```python
from build123d import *

# Parameters (mm, degrees)
SKETCH1_W           = 90
SKETCH1_H           = 50
BOSS_EXTRUDE1_DEPTH = 40
SKETCH21_R          = 5
CUT_EXTRUDE10_DEPTH = 40
SKETCH22_W          = 40
SKETCH22_H          = 13.4
CUT_EXTRUDE11_DEPTH = 9
SKETCH24_W          = 24
SKETCH24_H          = 13.4
CUT_EXTRUDE12_DEPTH = 31
SKETCH25_R          = 1.1
CUT_EXTRUDE13_DEPTH = 31
SKETCH31_W          = 25
SKETCH31_H          = 40
BOSS_EXTRUDE2_DEPTH = 50
SKETCH32_R          = 10
CUT_EXTRUDE15_DEPTH = 25
CHAMFER1_SIZE       = 10
CUT_EXTRUDE16_REACH = 142.357
SKETCH35_W          = 15
SKETCH35_H          = 20
SKETCH36_W          = 12
SKETCH36_H          = 12
SKETCH36_R          = 3.5
BOSS_EXTRUDE3_DEPTH = 10


with BuildPart() as part:
    # Sketch1 → Boss-Extrude1 (new body)
    with BuildSketch(Plane.XY):
        with Locations((-45, 25)):
            Rectangle(SKETCH1_W, SKETCH1_H)
    extrude(amount=BOSS_EXTRUDE1_DEPTH)

    # Sketch21 → Cut-Extrude10 (cut)
    with BuildSketch(Plane.XY.offset(40)):
        with Locations((-25, 25)):
            Circle(SKETCH21_R)
        with BuildLine():
            Line((-25, 30), (-30, 30))
            Line((-30, 30), (-30, 25))
            ThreePointArc((-30, 25), (-28.535533906, 28.535533906), (-25, 30))
        make_face()
        with BuildLine():
            ThreePointArc((-25, 20), (-28.535533906, 21.464466094), (-30, 25))
            Line((-30, 25), (-30, 20))
            Line((-30, 20), (-25, 20))
        make_face()
        with BuildLine():
            Line((-20, 20), (-20, 25))
            ThreePointArc((-20, 25), (-21.464466094, 21.464466094), (-25, 20))
            Line((-25, 20), (-20, 20))
        make_face()
        with BuildLine():
            Line((-20, 30), (-25, 30))
            ThreePointArc((-25, 30), (-21.464466094, 28.535533906), (-20, 25))
            Line((-20, 25), (-20, 30))
        make_face()
    extrude(amount=-CUT_EXTRUDE10_DEPTH, mode=Mode.SUBTRACT)

    # Sketch22 → Cut-Extrude11 (cut)
    with BuildSketch(Plane.XY.offset(40)):
        with Locations((-59.75, 25)):
            Rectangle(SKETCH22_W, SKETCH22_H)
    extrude(amount=-CUT_EXTRUDE11_DEPTH, mode=Mode.SUBTRACT)

    # Sketch24 → Cut-Extrude12 (cut)
    with BuildSketch(Plane.XY.offset(31)):
        with Locations((-59.75, 25)):
            Rectangle(SKETCH24_W, SKETCH24_H)
    extrude(amount=-CUT_EXTRUDE12_DEPTH, mode=Mode.SUBTRACT)

    # Sketch25 → Cut-Extrude13 (cut)
    with BuildSketch(Plane.XY.offset(31)):
        with Locations((-73.25, 25)):
            Circle(SKETCH25_R)
        with Locations((-46.25, 25)):
            Circle(SKETCH25_R)
    extrude(amount=-CUT_EXTRUDE13_DEPTH, mode=Mode.SUBTRACT)

    # Sketch31 → Boss-Extrude2 (add)
    with BuildSketch(Plane(origin=(0, 50, 0), x_dir=(1, 0, 0), z_dir=(0, 1, 0))):
        with Locations((-77.5, -20)):
            Rectangle(SKETCH31_W, SKETCH31_H)
    extrude(amount=BOSS_EXTRUDE2_DEPTH)

    # Sketch32 → Cut-Extrude15 (cut)
    with BuildSketch(Plane(origin=(-65, 0, 0), x_dir=(0, 0, -1), z_dir=(1, 0, 0))):
        with BuildLine():
            ThreePointArc((-40, 80), (-34.142135624, 94.142135624), (-20, 100))
            Line((-20, 100), (-40, 100))
            Line((-40, 100), (-40, 80))
        make_face()
        with BuildLine():
            ThreePointArc((-20, 100), (-5.857864376, 94.142135624), (0, 80))
            Line((0, 80), (0, 100))
            Line((0, 100), (-20, 100))
        make_face()
        with Locations((-20, 80)):
            Circle(SKETCH32_R)
    extrude(amount=-CUT_EXTRUDE15_DEPTH, mode=Mode.SUBTRACT)

    # Chamfer1
    chamfer1_edges = [part.edges().sort_by_distance(p)[0] for p in [
        (-65, 50, 20),
        (0, 50, 20),
        (0, 0, 20),
        (-90, 0, 20),
    ]]
    chamfer(chamfer1_edges, length=CHAMFER1_SIZE)

    # Cut-Extrude16: up to this face of the body (flat: up to its plane)
    cut_extrude16_end = Plane(part.part.faces().sort_by_distance((-47.75, 25, 15.5))[0])
    # Sketch35 → Cut-Extrude16 (cut, up to the picked face)
    with BuildSketch(Plane.ZY.offset(90), mode=Mode.PRIVATE) as cut_extrude16_sk1:
        with Locations((14.686432503, 25)):
            Rectangle(SKETCH35_W, SKETCH35_H)
    cut_extrude16_tool1 = split(extrude(cut_extrude16_sk1.sketch, amount=-CUT_EXTRUDE16_REACH, mode=Mode.PRIVATE), bisect_by=cut_extrude16_end, keep=Keep.BOTH, mode=Mode.PRIVATE)
    add(cut_extrude16_tool1.solids().sort_by(Axis((-90, 25, 14.686433), (1, 0, 0)))[0], mode=Mode.SUBTRACT)

    # Sketch36 → Boss-Extrude3 (add)
    # profile 1 of 2: a face of its own
    with BuildSketch(Plane.XY.offset(40)):
        with Locations((-65, -6)):
            Rectangle(SKETCH36_W, SKETCH36_H)
        with Locations((-65, -6)):
            Circle(SKETCH36_R, mode=Mode.SUBTRACT)
    # profile 2 of 2: a face of its own
    with BuildSketch(Plane.XY.offset(40)):
        with Locations((-25, -6)):
            Rectangle(SKETCH36_W, SKETCH36_H)
        with Locations((-25, -6)):
            Circle(SKETCH36_R, mode=Mode.SUBTRACT)
    extrude(amount=-BOSS_EXTRUDE3_DEPTH)


solid = part.part
```
Work out the finished part from the listing and answer in its coordinate system (mm). A direction names the side the tool comes from. Coordinates: 2 decimals unless noted, no trailing zeros. Write each loop counter-clockwise with the first axis right and the second up, starting at its lowest first coordinate (ties: lowest second). Pieces come first, ordered by that corner, then holes.
Q1. Determine the mould class of faces 1 (the face through (-47.75, 25, 16)), 2 (the face through (-85, 5, 20)), 3 (the face through (-25, -12, 35)) for opening direction X: released by +X, released by -X, zero draft, split by the parting line, or undercut.
Q2. Find the intervals of material crossed by line 1 (Y direction, x = -72, z = 20); line 2 (Y direction, x = -22, z = 14); line 3 (Y direction, x = -54.5, z = 23), in increasing order.
Q3. Each of these flat-tipped pins is pushed along its axis until it touches: pin 1 Ø12 at (y, z) = (59.5, 13.5) entering from +X; pin 2 Ø5.5 at (x, z) = (-50.5, 30) entering from +Y; pin 3 Ø4 at (y, z) = (50, 32.5) entering from +X; pin 4 Ø2 at (x, y) = (-73.25, 25) entering from +Z. Where does it stop, or does it pass through?
Q4. Which of the six approach directions +Z, -Z, +X, -X, +Y, -Y give full straight-line access (tool end or side, diameter ignored) to faces 4 (the face through (-19, -6, 35)), 5 (the face through (-65, 71, 25)), 6 (the face through (-71.75, 25, 27)), 7 (the face through (-74, 23, 7.186)), 8 (the face through (-22, -3, 30))?
Q5. A cutting plane is placed at B-B, the plane z = 24.5. Give the vertices of the cut face in (x, y), then the cut area to 3 significant figures.
Q6. A cutting plane is placed at C-C, the plane x = -25. Give the vertices of the cut face in (y, z).
Q7. A cutting plane is placed at D-D, the plane z = 34.5. Give the vertices of the cut face in (x, y).
Q8. A cutting plane is placed at A-A, the plane x = -51.5. Give the vertices of the cut face in (y, z), then the cut area to 4 significant figures.
Findings below:
1. face 1: undercut
1. face 2: released by -X
1. face 3: zero draft
2. line 1: y = 0 to 15, 35 to 70, 90 to 100
2. line 2: y = 0 to 20, 30 to 50
2. line 3: y = 0 to 18.3, 31.7 to 50
3. pin 1: stops at x = -58.5
3. pin 2: stops at y = 50
3. pin 3: stops at x = -8
3. pin 4: passes through
4. face 4: +Z, -Z, +X, -Y
4. face 5: +Z, -Z, +X, +Y
4. face 6: +Z, -Z
4. face 7: -X
4. face 8: -Z, +X, -X, -Y
5. outline: (-90, 10) - (-80, 0) - (-10, 0) - (0, 10) - (0, 40) - (-10, 50) - (-55, 50) - (-65, 60) - (-65, 71.07) - (-90, 71.07) - close; (-90, 88.93) - (-65, 88.93) - (-65, 99.49) - (-90, 99.49) - close; hole circle Ø2.2 at (-73.25, 25); hole (-71.75, 18.3) - (-47.75, 18.3) - (-47.75, 31.7) - (-71.75, 31.7) - close; hole circle Ø2.2 at (-46.25, 25); hole (-30, 20) - (-20, 20) - (-20, 30) - (-30, 30) - close
5. area: 4,760 mm2
6. outline: (-12, 30) - (-9.5, 30) - (-9.5, 40) - (-12, 40) - close; (-2.5, 30) - (0, 30) - (0, 0) - (20, 0) - (20, 40) - (-2.5, 40) - close; (30, 0) - (50, 0) - (50, 40) - (30, 40) - close
7. outline: (-90, 10) - (-80, 0) - (-71, 0) - (-71, -12) - (-59, -12) - (-59, 0) - (-31, 0) - (-31, -12) - (-19, -12) - (-19, 0) - (-10, 0) - (0, 10) - (0, 40) - (-10, 50) - (-55, 50) - (-65, 60) - (-65, 93.77) - (-90, 93.77) - close; hole (-79.75, 18.3) - (-39.75, 18.3) - (-39.75, 31.7) - (-79.75, 31.7) - close; hole circle Ø7 at (-65, -6); hole (-30, 20) - (-20, 20) - (-20, 30) - (-30, 30) - close; hole circle Ø7 at (-25, -6)
8. outline: (0, 0) - (18.3, 0) - (18.3, 7.19) - (15, 7.19) - (15, 22.19) - (18.3, 22.19) - (18.3, 40) - (0, 40) - close; (31.7, 0) - (50, 0) - (50, 40) - (31.7, 40) - (31.7, 22.19) - (35, 22.19) - (35, 7.19) - (31.7, 7.19) - close
8. area: 1,365 mm2
